Part print with two shaded views. Sizes in mm from the minimum x, y, z corner. A direction names the side the tool comes from. Give positions to 0.01 mm unless a question says otherwise; leave off trailing zeros. Write each loop counter-clockwise with the first axis right and the second up, starting at its lowest first coordinate (ties: lowest second). Pieces come first, ordered by that corner, then holes. Notation, with made-up numbers: (-18, -36.5) -> (2, -36.5) arc R26 ccw to (2, -3.5) -> close; hole circle Ø9 at (-17.75, 72). An arc over 180 degrees is marked (long way). Answer as a JSON object with one key per item and string values.
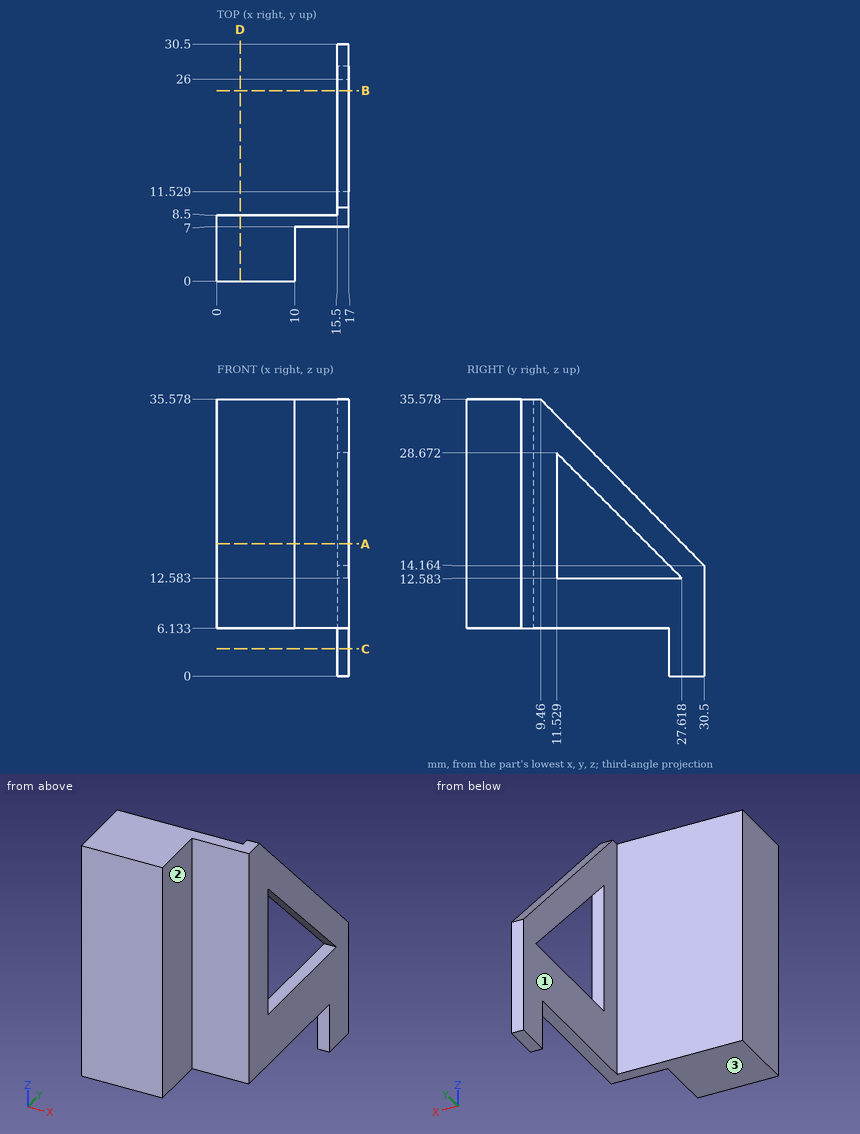
1) Slice it at B-B (y = 24.5). List the corners of the cut face in (x, z).
Model answer:
{"outline": "(15.5, 6.13) -> (17, 6.13) -> (17, 12.58) -> (15.5, 12.58) -> close; (15.5, 15.7) -> (17, 15.7) -> (17, 20.27) -> (15.5, 20.27) -> close"}
2) Slice it at D-D (x = 3). List the corners of the cut face in (y, z), then the cut area to 3 significant figures.
Model answer:
{"outline": "(0, 6.13) -> (8.5, 6.13) -> (8.5, 35.58) -> (0, 35.58) -> close", "area": "250 mm2"}
3) Pin check, flat tips, straight feed: pin 1 (8 mm diameter, centred on x = 6, y = 5, fed in from -Z); pin 2 (2 mm diameter, centred on y = 3.5, z = 25.5, fed in from +X); pin 3 (5.5 mm diameter, centred on x = 14, z = 23, fed in from -Y). Stop position of each tip, or through.
Model answer:
{"pin 1": "stops at z = 6.13", "pin 2": "stops at x = 10", "pin 3": "stops at y = 7"}
4) Wall check: probe 1 along Z at (x, y) = (2.5, 7); probe 2 along Y at (x, z) = (7.5, 12.5); probe 3 along X at (y, z) = (3, 13). Give the ranges that are in metal, low to high.
Model answer:
{"probe 1": "z = 6.13 to 35.58", "probe 2": "y = 0 to 8.5", "probe 3": "x = 0 to 10"}
5) Slice it at C-C (z = 3.5). List the corners of the cut face in (x, y).
Model answer:
{"outline": "(15.5, 26) -> (17, 26) -> (17, 30.5) -> (15.5, 30.5) -> close"}
6) Slice it at A-A (z = 17). List the corners of the cut face in (x, y).
Model answer:
{"outline": "(0, 0) -> (10, 0) -> (10, 7) -> (17, 7) -> (17, 11.53) -> (15.5, 11.53) -> (15.5, 8.5) -> (0, 8.5) -> close; (15.5, 23.2) -> (17, 23.2) -> (17, 27.71) -> (15.5, 27.71) -> close"}
7) 3-axis set-ups, long thin cutter, end or side, ignore diameter. For the marked faces 1, 2 and 3: which of +Z, -Z, +X, -X, +Y, -Y reach the whole face in a straight line?
Model answer:
{"face 1": "+Z, -Z, -X, +Y", "face 2": "+Z, -Z, +X, -Y", "face 3": "-Z, +X, -X, -Y"}
